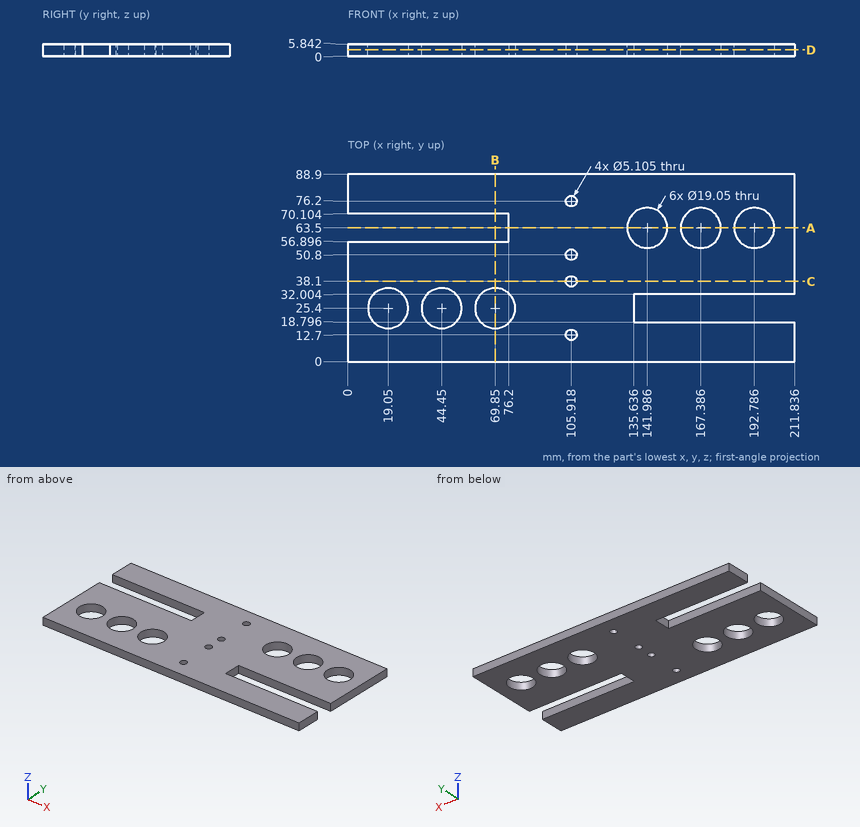
Here's the drawing with two shaded views (mm, measured from the low corner). I have some questions. Coordinates: 2 decimals unless noted, no trailing zeros. Write each loop counter-clockwise with the first axis right and the second up, starting at its lowest first coordinate (ties: lowest second). Pieces come first, ordered by that corner, then holes.
Item 1: I want a section at A-A on y = 63.5. Write out the boundary of the cut face in (x, z).
Item 2: I want a section at B-B on x = 69.85. Write out the boundary of the cut face in (y, z) (1 decimal), and give its area (3 significant figures).
Item 3: I want a section at C-C on y = 38.1. Write out the boundary of the cut face in (x, z) (1 decimal).
Item 4: I want a section at D-D on z = 3.05. Count the separate pieces of the cut face and the enclosed holes in it, and give its area (3 significant figures).
Item 5: If I drill on line 1 (Y direction, x = 69.85, z = 3.3) (1 decimal); line 2 (X direction, y = 25.5, z = 0.65) (1 decimal); line 3 (X direction, y = 61.5, z = 4.75) (1 decimal), over which ranges is the centre line in solid material (lowest first)?
Item 6: Will these pins go through, and if not, where does the flat tip stop? pin 1 (2 mm diameter, centred on y = 20, z = 0.5, fed in from +X); pin 2 (1.8 mm diameter, centred on y = 62.5, z = 3, fed in from -X).
Findings below:
1. outline: (76.2, 0) - (132.46, 0) - (132.46, 5.84) - (76.2, 5.84) - close; (151.51, 0) - (157.86, 0) - (157.86, 5.84) - (151.51, 5.84) - close; (176.91, 0) - (183.26, 0) - (183.26, 5.84) - (176.91, 5.84) - close; (202.31, 0) - (211.84, 0) - (211.84, 5.84) - (202.31, 5.84) - close
2. outline: (0, 0) - (15.9, 0) - (15.9, 5.8) - (0, 5.8) - close; (34.9, 0) - (56.9, 0) - (56.9, 5.8) - (34.9, 5.8) - close; (70.1, 0) - (88.9, 0) - (88.9, 5.8) - (70.1, 5.8) - close
2. area: 331 mm2
3. outline: (0, 0) - (103.4, 0) - (103.4, 5.8) - (0, 5.8) - close; (108.5, 0) - (211.8, 0) - (211.8, 5.8) - (108.5, 5.8) - close
4. separate pieces: 1
4. enclosed holes: 10
4. area: 15,000 mm2
5. line 1: y = 0 to 15.9, 34.9 to 56.9, 70.1 to 88.9
5. line 2: x = 0 to 9.5, 28.6 to 34.9, 54 to 60.3, 79.4 to 135.6
5. line 3: x = 76.2 to 132.7, 151.3 to 158.1, 176.7 to 183.5, 202.1 to 211.8
6. pin 1: stops at x = 135.64
6. pin 2: stops at x = 76.2
